Check sheet for the modelled part. Datum: model origin and axes. Units: mm. Give positions to 0.01 mm unless a question says otherwise; leave off trailing zeros. Answer as CSV lines item,"result". Start each with the question number.
(1) Release check for a two-part mould opening along X. For faces 1 (the face through (0, 301, -25)), 2 (the face through (25, 606.425, -26)), 3 (the face through (8, 609.6, -25)) record: pulls with the +X half, pulls with the -X half, needs draft (parallel to the pull), parting line crosses it, or undercut.
(2) Material ranges on line 1 (Y direction, x = 22, z = -25.5) (3 decimals), recorded low to high. Write a range as from..to.
(3) Gauge pin test, flat end, axial feed: pin 1 Ø12.5 at (x, z) = (27.5, -30) entering from +Y (3 decimals). Record the tip position at first contact, or that the pin passes through.
Autodesk Inventor part; units mm, degrees
ref_plane "YZ Plane" through (0, 0, 0) normal (1, 0, 0) x (0, 1, 0)
ref_plane "XZ Plane" through (0, 0, 0) normal (0, 1, 0) x (-1, 0, 0)
ref_plane "XY Plane" through (0, 0, 0) normal (0, 0, 1) x (1, 0, 0)
sketch "Sketch1" plane through (0, 0, 0) normal (1, 0, 0) x (0, 1, 0)
  line L0 (0, 0) -> (609.6, 0)
  line L1 (609.6, 0) -> (609.6, -50.8)
  line L2 (609.6, -50.8) -> (0, -50.8)
  line L3 (0, -50.8) -> (0, 0)
  dimension "d0" = 609.6
  dimension "d1" = 50.8
extrude "Extrusion1" add sketch "Sketch1" along normal blind 50.8
sketch "Sketch2" plane through (0, 609.6, 0) normal (0, 1, 0) x (1, 0, 0)
  line L0 (12.7, 38.1) -> (38.1, 38.1)
  line L1 (38.1, 38.1) -> (38.1, 12.7)
  line L2 (38.1, 12.7) -> (12.7, 12.7)
  line L3 (12.7, 12.7) -> (12.7, 38.1)
  line L4 (0, 0) -> (0, 50.8)
  line L5 (0, 50.8) -> (50.8, 50.8)
  dimension "d4" = 25.4
  dimension "d5" = 25.4
  dimension "d6" = 12.7
  dimension "d7" = 12.7
extrude "Extrusion2" cut sketch "Sketch2" against normal blind 3.175
properties part number "LegStandard" material "Wood (Birch)"
Working result:
1,face 1,"pulls with the -X half"
1,face 2,"undercut"
1,face 3,"needs draft"
2,line 1,"y = 0..606.425"
3,pin 1,"stops at y = 606.425"
